from build123d import *

# Parameters (mm, degrees)
SKETCH_1_W           = 30
SKETCH_1_H           = 40
SKETCH_1_W_2         = 28
SKETCH_1_H_2         = 38
EXTRUDE_1_DEPTH      = 1000
SKETCH_2_R           = 1.6
CUT_EXTRUDE_1_DEPTH  = 10
SKETCH_3_R           = 1.6
CUT_EXTRUDE_2_DEPTH  = 1001.912084051
SKETCH_5_R           = 2.6
CUT_EXTRUDE_3_DEPTH  = 1001.912084051
SKETCH_6_R           = 2.05
CUT_EXTRUDE_4_DEPTH  = 1
SKETCH_7_R           = 1.6
CUT_EXTRUDE_5_DEPTH  = 1
SKETCH_9_R           = 3
CUT_EXTRUDE_9_DEPTH  = 1
SKETCH_11_R          = 1.6
CUT_EXTRUDE_10_DEPTH = 1001.912084051
SKETCH_12_R          = 3.25
CUT_EXTRUDE_11_DEPTH = 1
SKETCH_16_R          = 3
CUT_EXTRUDE_15_DEPTH = 1
SKETCH_18_R          = 1.55
CUT_EXTRUDE_16_DEPTH = 10
SKETCH_21_R          = 1.6
CUT_EXTRUDE_18_DEPTH = 1001.912084051
SKETCH_23_R          = 1.55
CUT_EXTRUDE_19_DEPTH = 30


with BuildPart() as part:
    # 草图1 → 凸台-拉伸1 (new body)
    with BuildSketch(Plane.XY):
        Rectangle(SKETCH_1_W, SKETCH_1_H)
        Rectangle(SKETCH_1_W_2, SKETCH_1_H_2, mode=Mode.SUBTRACT)
    extrude(amount=EXTRUDE_1_DEPTH)

    # 草图2 → 切除-拉伸1 (cut)
    with BuildSketch(Plane(origin=(15, 0, 0), x_dir=(0, 0, -1), z_dir=(1, 0, 0))):
        with Locations((-995, 14)):
            Circle(SKETCH_2_R)
        with Locations((-995, -14)):
            Circle(SKETCH_2_R)
        with Locations((-5, 14)):
            Circle(SKETCH_2_R)
        with Locations((-5, -14)):
            Circle(SKETCH_2_R)
    extrude(amount=-CUT_EXTRUDE_1_DEPTH, mode=Mode.SUBTRACT)

    # 草图3 → 切除-拉伸2 (cut, through all)
    with BuildSketch(Plane(origin=(0, 20, 0), x_dir=(1, 0, 0), z_dir=(0, 1, 0))):
        with Locations(Location((-9, -995, 0), (0, 0, 270))):
            Circle(SKETCH_3_R)
        with Locations(Location((-9, -5, 0), (0, 0, 270))):
            Circle(SKETCH_3_R)
    extrude(amount=-CUT_EXTRUDE_2_DEPTH, mode=Mode.SUBTRACT)

    # 草图5 → 切除-拉伸3 (cut, through all)
    with BuildSketch(Plane.XZ.offset(20)):
        with Locations(Location((-8, 53, 0), (0, 0, 270))):
            Circle(SKETCH_5_R)
        with Locations(Location((8, 53, 0), (0, 0, 270))):
            Circle(SKETCH_5_R)
        with Locations(Location((-8, 97, 0), (0, 0, 270))):
            Circle(SKETCH_5_R)
        with Locations(Location((8, 97, 0), (0, 0, 270))):
            Circle(SKETCH_5_R)
    extrude(amount=-CUT_EXTRUDE_3_DEPTH, mode=Mode.SUBTRACT)

    # 草图6 → 切除-拉伸4 (cut)
    with BuildSketch(Plane(origin=(15, 0, 0), x_dir=(0, 0, -1), z_dir=(1, 0, 0))):
        with Locations((-40, 15)):
            Circle(SKETCH_6_R)
        with Locations((-15, 15)):
            Circle(SKETCH_6_R)
        with Locations((-15, -15)):
            Circle(SKETCH_6_R)
        with Locations((-40, -15)):
            Circle(SKETCH_6_R)
        with BuildLine():
            Line((-345, -7.5), (-375, -7.5))
            ThreePointArc((-375, -7.5), (-382.5, 0), (-375, 7.5))
            Line((-375, 7.5), (-345, 7.5))
            ThreePointArc((-345, 7.5), (-337.5, 0), (-345, -7.5))
        make_face()
        with BuildLine():
            Line((-595, -7.5), (-625, -7.5))
            ThreePointArc((-625, -7.5), (-632.5, 0), (-625, 7.5))
            Line((-625, 7.5), (-595, 7.5))
            ThreePointArc((-595, 7.5), (-587.5, 0), (-595, -7.5))
        make_face()
        with BuildLine():
            Line((-815, -7.5), (-845, -7.5))
            ThreePointArc((-845, -7.5), (-852.5, 0), (-845, 7.5))
            Line((-845, 7.5), (-815, 7.5))
            ThreePointArc((-815, 7.5), (-807.5, 0), (-815, -7.5))
        make_face()
    extrude(amount=-CUT_EXTRUDE_4_DEPTH, mode=Mode.SUBTRACT)

    # 草图7 → 切除-拉伸5 (cut)
    with BuildSketch(Plane.ZY.offset(15)):
        with Locations((350, 0)):
            Circle(SKETCH_7_R)
        with Locations((370, 0)):
            Circle(SKETCH_7_R)
        with Locations((600, 0)):
            Circle(SKETCH_7_R)
        with Locations((620, 0)):
            Circle(SKETCH_7_R)
        with Locations((850, 0)):
            Circle(SKETCH_7_R)
        with Locations((870, 0)):
            Circle(SKETCH_7_R)
    extrude(amount=-CUT_EXTRUDE_5_DEPTH, mode=Mode.SUBTRACT)

    # 草图9 → 切除-拉伸9 (cut)
    with BuildSketch(Plane(origin=(0, 20, 0), x_dir=(1, 0, 0), z_dir=(0, 1, 0))):
        with Locations(Location((-10, -507.5, 0), (0, 0, 270))):
            Circle(SKETCH_9_R)
        with Locations(Location((-10, -497.5, 0), (0, 0, 270))):
            Circle(SKETCH_9_R)
        with Locations(Location((10, -497.5, 0), (0, 0, 270))):
            Circle(SKETCH_9_R)
        with Locations(Location((10, -507.5, 0), (0, 0, 270))):
            Circle(SKETCH_9_R)
        with Locations(Location((-10, -147.5, 0), (0, 0, 270))):
            Circle(SKETCH_9_R)
        with Locations(Location((-10, -157.5, 0), (0, 0, 270))):
            Circle(SKETCH_9_R)
        with Locations(Location((10, -157.5, 0), (0, 0, 270))):
            Circle(SKETCH_9_R)
        with Locations(Location((10, -147.5, 0), (0, 0, 270))):
            Circle(SKETCH_9_R)
    extrude(amount=-CUT_EXTRUDE_9_DEPTH, mode=Mode.SUBTRACT)

    # 草图11 → 切除-拉伸10 (cut, through all)
    with BuildSketch(Plane(origin=(0, 20, 0), x_dir=(1, 0, 0), z_dir=(0, 1, 0))):
        with Locations(Location((-7, -177.5, 0), (0, 0, 270))):
            Circle(SKETCH_11_R)
        with Locations(Location((7, -177.5, 0), (0, 0, 270))):
            Circle(SKETCH_11_R)
        with Locations(Location((-7, -227.5, 0), (0, 0, 270))):
            Circle(SKETCH_11_R)
        with Locations(Location((7, -227.5, 0), (0, 0, 270))):
            Circle(SKETCH_11_R)
        with Locations(Location((-7, -277.5, 0), (0, 0, 270))):
            Circle(SKETCH_11_R)
        with Locations(Location((7, -277.5, 0), (0, 0, 270))):
            Circle(SKETCH_11_R)
        with Locations(Location((-7, -327.5, 0), (0, 0, 270))):
            Circle(SKETCH_11_R)
        with Locations(Location((7, -327.5, 0), (0, 0, 270))):
            Circle(SKETCH_11_R)
        with Locations(Location((-7, -377.5, 0), (0, 0, 270))):
            Circle(SKETCH_11_R)
        with Locations(Location((7, -377.5, 0), (0, 0, 270))):
            Circle(SKETCH_11_R)
        with Locations(Location((-7, -427.5, 0), (0, 0, 270))):
            Circle(SKETCH_11_R)
        with Locations(Location((7, -427.5, 0), (0, 0, 270))):
            Circle(SKETCH_11_R)
    extrude(amount=-CUT_EXTRUDE_10_DEPTH, mode=Mode.SUBTRACT)

    # 草图12 → 切除-拉伸11 (cut)
    with BuildSketch(Plane.XZ.offset(20)):
        with Locations(Location((-7, 227.5, 0), (0, 0, 270))):
            Circle(SKETCH_12_R)
        with Locations(Location((7, 227.5, 0), (0, 0, 270))):
            Circle(SKETCH_12_R)
        with Locations(Location((-7, 277.5, 0), (0, 0, 270))):
            Circle(SKETCH_12_R)
        with Locations(Location((7, 277.5, 0), (0, 0, 270))):
            Circle(SKETCH_12_R)
        with Locations(Location((-7, 327.5, 0), (0, 0, 270))):
            Circle(SKETCH_12_R)
        with Locations(Location((-7, 177.5, 0), (0, 0, 270))):
            Circle(SKETCH_12_R)
        with Locations(Location((7, 177.5, 0), (0, 0, 270))):
            Circle(SKETCH_12_R)
        with Locations(Location((7, 327.5, 0), (0, 0, 270))):
            Circle(SKETCH_12_R)
        with Locations(Location((-7, 377.5, 0), (0, 0, 270))):
            Circle(SKETCH_12_R)
        with Locations(Location((7, 377.5, 0), (0, 0, 270))):
            Circle(SKETCH_12_R)
        with Locations(Location((-7, 427.5, 0), (0, 0, 270))):
            Circle(SKETCH_12_R)
        with Locations(Location((7, 427.5, 0), (0, 0, 270))):
            Circle(SKETCH_12_R)
    extrude(amount=-CUT_EXTRUDE_11_DEPTH, mode=Mode.SUBTRACT)

    # 草图16 → 切除-拉伸15 (cut)
    with BuildSketch(Plane(origin=(0, 20, 0), x_dir=(1, 0, 0), z_dir=(0, 1, 0))):
        with Locations(Location((-7, -770, 0), (0, 0, 270))):
            Circle(SKETCH_16_R)
        with Locations(Location((7, -770, 0), (0, 0, 270))):
            Circle(SKETCH_16_R)
        with Locations(Location((-7, -590, 0), (0, 0, 270))):
            Circle(SKETCH_16_R)
        with Locations(Location((-7, -746, 0), (0, 0, 270))):
            Circle(SKETCH_16_R)
        with Locations(Location((7, -590, 0), (0, 0, 270))):
            Circle(SKETCH_16_R)
        with Locations(Location((7, -746, 0), (0, 0, 270))):
            Circle(SKETCH_16_R)
        with Locations(Location((7, -566, 0), (0, 0, 270))):
            Circle(SKETCH_16_R)
        with Locations(Location((-7, -566, 0), (0, 0, 270))):
            Circle(SKETCH_16_R)
    extrude(amount=-CUT_EXTRUDE_15_DEPTH, mode=Mode.SUBTRACT)

    # 草图18 → 切除-拉伸16 (cut)
    with BuildSketch(Plane.XZ.offset(20)):
        with Locations(Location((-7, 770, 0), (0, 0, 270))):
            Circle(SKETCH_18_R)
        with Locations(Location((7, 770, 0), (0, 0, 270))):
            Circle(SKETCH_18_R)
        with Locations(Location((-7, 746, 0), (0, 0, 270))):
            Circle(SKETCH_18_R)
        with Locations(Location((7, 746, 0), (0, 0, 270))):
            Circle(SKETCH_18_R)
    extrude(amount=-CUT_EXTRUDE_16_DEPTH, mode=Mode.SUBTRACT)

    # 草图21 → 切除-拉伸18 (cut, through all)
    with BuildSketch(Plane.XZ.offset(20)):
        with Locations(Location((-10, 147.5, 0), (0, 0, 270))):
            Circle(SKETCH_21_R)
        with Locations(Location((-10, 157.5, 0), (0, 0, 270))):
            Circle(SKETCH_21_R)
        with Locations(Location((10, 147.5, 0), (0, 0, 270))):
            Circle(SKETCH_21_R)
        with Locations(Location((10, 157.5, 0), (0, 0, 270))):
            Circle(SKETCH_21_R)
        with Locations(Location((-10, 497.5, 0), (0, 0, 270))):
            Circle(SKETCH_21_R)
        with Locations(Location((-10, 507.5, 0), (0, 0, 270))):
            Circle(SKETCH_21_R)
        with Locations(Location((10, 497.5, 0), (0, 0, 270))):
            Circle(SKETCH_21_R)
        with Locations(Location((10, 507.5, 0), (0, 0, 270))):
            Circle(SKETCH_21_R)
        with Locations(Location((-7, 566, 0), (0, 0, 270))):
            Circle(SKETCH_21_R)
        with Locations(Location((-7, 590, 0), (0, 0, 270))):
            Circle(SKETCH_21_R)
        with Locations(Location((7, 566, 0), (0, 0, 270))):
            Circle(SKETCH_21_R)
        with Locations(Location((7, 590, 0), (0, 0, 270))):
            Circle(SKETCH_21_R)
        with Locations(Location((-7, 746, 0), (0, 0, 270))):
            Circle(SKETCH_21_R)
        with Locations(Location((-7, 770, 0), (0, 0, 270))):
            Circle(SKETCH_21_R)
        with Locations(Location((7, 746, 0), (0, 0, 270))):
            Circle(SKETCH_21_R)
        with Locations(Location((7, 770, 0), (0, 0, 270))):
            Circle(SKETCH_21_R)
    extrude(amount=-CUT_EXTRUDE_18_DEPTH, mode=Mode.SUBTRACT)

    # 草图23 → 切除-拉伸19 (cut)
    with BuildSketch(Plane(origin=(15, 0, 0), x_dir=(0, 0, -1), z_dir=(1, 0, 0))):
        with Locations((-116, 10)):
            Circle(SKETCH_23_R)
        with Locations((-116, -10)):
            Circle(SKETCH_23_R)
    extrude(amount=-CUT_EXTRUDE_19_DEPTH, mode=Mode.SUBTRACT)


solid = part.part
Design review of the part built by this model. Coordinates are the model's own, in mm. A direction names the side the tool comes from. Round coordinates to 2 decimals unless told otherwise and drop trailing zeros. Order: outer loops, then holes, each group sorted by start corner. A loop starts at its lowest first (then second) coordinate and runs counter-clockwise, first axis right, second up. Notation, with made-up numbers: M 43.25,-11 L 90.25,-11 A23 cw 90.25,19 Z; hole C 35.5,17.25 d11. An arc over 180 degrees is marked long. Answer as CSV lines item,"result". Start each with the question number.
1) For pin 1 Ø4 at (y, z) = (0, 620) entering from +X; pin 2 Ø5 at (x, z) = (7, 377.5) entering from -Y, all flat-tipped, find the tip position at first contact; note any pin that passes through.
2) Tool access review of faces 1 (the face through (0, -19, 493)), 2 (the face through (0, 20, 493)): name each direction out of +Z, -Z, +X, -X, +Y, -Y from which nothing blocks a thin tool from reaching the whole face with its end or side.
3) Wall thickness on line 1 along X through (y, z) = (-19.8, 497.5); line 2 along X through (y, z) = (3, 56); line 3 along X through (y, z) = (-19.6, 377.5): over which ranges is each line inside the solid? List them lowest first. Write a range as [from, to].
4) Add section A-A (z = 306). Give the boundary of the cut face in (x, y), then the cut area to 3 significant figures.
5) The part is to be moulded in two halves that separate along X. For faces 3 (the face through (15, 0, 493)), 4 (the face through (0, 19, 493)), 5 (the face through (-14.5, 0.1, 1000)), say which applies: +X half, -X half, draft (parallel to the pull), parting line (faces both ways), or undercut.
Resolved:
1,pin 1,"x = -14"
1,pin 2,"y = 19"
2,face 1,"+Z, -Z"
2,face 2,"+Z, -Z, +X, -X, +Y"
3,line 1,"[-15, -11.6], [-8.4, 8.4], [11.6, 15]"
3,line 2,"[-15, -14], [14, 15]"
3,line 3,"[-15, -10.25], [-3.75, 3.75], [10.25, 15]"
4,outline,"M -15,-20 L 15,-20 L 15,20 L -15,20 Z; hole M -14,-19 L 14,-19 L 14,19 L -14,19 Z"
4,area,"136 mm^2"
5,face 3,"+X half"
5,face 4,"undercut"
5,face 5,"draft"
